```python
from build123d import *

# Parameters (mm, degrees)
F0_R     = 37.1794953158
F1_DEPTH = 73.66
F3_DEPTH = 67.818
F4_R     = 24.1009432371
F5_DEPTH = 73.914


with BuildPart() as f1:
    # F0 (on Top) → F1 (new body)
    with BuildSketch(Plane.XY):
        with Locations((0, 4.0802885778)):
            Circle(F0_R)
    extrude(amount=F1_DEPTH)

    # F2 (on face) + F0 (on Top) → F3 (join)
    with BuildSketch(Plane.XY):
        with BuildLine():
            Line((-17.3161878706, 36.9811169803), (-67.2493875027, 36.9811169803))
            Line((-67.2493875027, 36.9811169803), (-67.2493875027, -48.5952086747))
            Line((-67.2493875027, -48.5952086747), (51.5947751701, -48.5952086747))
            Line((51.5947751701, -48.5952086747), (51.5947751701, 36.9811169803))
            Line((51.5947751701, 36.9811169803), (17.3161878706, 36.9811169803))
            ThreePointArc((17.3161878706, 36.9811169803), (31.8286191796, 23.2962682057), (37.1794953158, 4.0802885778))
            ThreePointArc((37.1794953158, 4.0802885778), (-19.2159796279, -27.7483306018), (-17.3161878706, 36.9811169803))
        make_face()
    with BuildSketch(Plane.XY):
        with Locations((0, 4.0802885778)):
            Circle(F0_R)
    extrude(amount=-F3_DEPTH)

    # F4 (on face) → F5 (join)
    with BuildSketch(Plane.XZ.offset(48.5952086747)):
        with Locations((-22.2101341933, -32.9192616045)):
            Circle(F4_R)
    extrude(amount=F5_DEPTH)


solid = f1.part
```
For this review, take the finished solid that the model builds, in its own axes (mm). A direction names the side the tool comes from. Give positions to 0.01 mm unless a question says otherwise; leave off trailing zeros. Write each loop counter-clockwise with the first axis right and the second up, starting at its lowest first coordinate (ties: lowest second). Pieces come first, ordered by that corner, then holes. Notation, with made-up numbers: M 23.25,-1.5 L 51.25,-1.5 A35 cw 51.25,35.5 Z; hole C 7,48.5 d6. An arc over 180 degrees is marked long. One line per item, written item: value.
1) Take a section at C-C, the plane z = 51. Write out the cut boundary in (x, y).
Results are:
outline: C 0,4.08 d74.36
2) Take a section at B-B, the plane y = -31. Write out the cut boundary in (x, z).
Results are:
outline: M -67.25,-67.82 L 51.59,-67.82 L 51.59,0 L 12.32,0 L 12.32,73.66 L -12.32,73.66 L -12.32,0 L -67.25,0 Z
3) For line 1 (Z direction, x = 33.5, y = 29); line 2 (Y direction, x = -52, z = -22); line 3 (Z direction, x = -23, y = -106.5), list the stretches that pass through material, from the lowest coordinate up. Write a range as from..to.
Results are:
line 1: z = -67.82..0
line 2: y = -48.6..36.98
line 3: z = -57.01..-8.83
4) Take a section at A-A, the plane x = 27. Write out the cut boundary in (y, z), then the cut area to 3 significant figures.
Results are:
outline: M -48.6,-67.82 L 36.98,-67.82 L 36.98,0 L 29.64,0 L 29.64,73.66 L -21.48,73.66 L -21.48,0 L -48.6,0 Z
area: 9,570 mm²
5) Take a section at D-D, the plane x = -1.5. Write out the cut boundary in (y, z), then the cut area to 3 significant figures.
Results are:
outline: M -122.51,-45.25 L -48.6,-45.25 L -48.6,-67.82 L 41.23,-67.82 L 41.23,73.66 L -33.07,73.66 L -33.07,0 L -48.6,0 L -48.6,-20.59 L -122.51,-20.59 Z
area: 13,400 mm²
6) For P1, Ø10, axis at y = 22.5, z = 57, coming from the +X side; P2, Ø3, axis at x = 1, y = -62, coming from the -Z side; P3, Ø1.5, axis at x = 9.5, z = -10.5, coming from the -Y side; P4, Ø6, axis at x = 7.5, y = -102.5, coming from the +Z side, all flat-tipped, find the tip position at first contact; note any pin that passes through.
Results are:
P1: stops at x = 34.67
P2: stops at z = -43.38
P3: stops at y = -48.6
P4: passes through
7) For faces 1 (the flat face through (35, 36.981, -33)), 2 (the flat face through (-23, -122.509, -33)), 3 (the flat face through (-1, 5, 73.66)), 4 (the flat face through (-42, 36.981, -33)), 5 (the cylindrical face through (0.778, -85.035, -25.68)), list the 3-axis set-ups (+Z, -Z, +X, -X, +Y, -Y) from which the entire face can be reached by the end or side of a thin tool; tool diameter is ignored.
Results are:
face 1: +Z, -Z, +X, +Y
face 2: +Z, -Z, +X, -X, -Y
face 3: +Z, +X, -X, +Y, -Y
face 4: +Z, -Z, -X, +Y
face 5: -Y
